Part model, mm, in its own coordinate system. A direction names the side the tool comes from. Round coordinates to 2 decimals unless told otherwise and drop trailing zeros. Answer as a JSON object with one key per item and string values. Group by question number.
from build123d import *

# Parameters (mm, degrees)
BOSS_EXTRUDE1_DEPTH = 4
BOSS_EXTRUDE1_TAPER = 10
CUT_EXTRUDE1_START  = 4
SKETCH1_3_R         = 1.1
CUT_EXTRUDE1_DEPTH  = 4
CUT_EXTRUDE2_START  = 4
SKETCH1_4_R         = 8.4
CUT_EXTRUDE2_DEPTH  = 3


with BuildPart() as part:
    # Sketch1 → Boss-Extrude1 (new body)
    with BuildSketch(Plane(origin=(0, 0, 0), x_dir=(1, 0, 0), z_dir=(0, 1, 0))):
        with BuildLine():
            ThreePointArc((-19.772689603, -11.447302995), (-15.6, -27.019992598), (-0.027310397, -22.847302995))
            Line((-0.027310397, -22.847302995), (9.872689603, -5.7))
            ThreePointArc((9.872689603, -5.7), (5.7, 9.872689603), (-9.872689603, 5.7))
            Line((-9.872689603, 5.7), (-19.772689603, -11.447302995))
        make_face()
    extrude(amount=BOSS_EXTRUDE1_DEPTH, taper=BOSS_EXTRUDE1_TAPER)

    # Sketch1<3> → Cut-Extrude1 (cut)
    with BuildSketch(Plane(origin=(0, 0, 0), x_dir=(1, 0, 0), z_dir=(0, 1, 0)).offset(CUT_EXTRUDE1_START)):
        with Locations(Location((-9.9, -17.147302995, 0), (0, 0, 270))):
            Circle(SKETCH1_3_R)
        with Locations(Location((0, 0, 0), (0, 0, 270))):
            Circle(SKETCH1_3_R)
    extrude(amount=-CUT_EXTRUDE1_DEPTH, mode=Mode.SUBTRACT)

    # Sketch1<4> → Cut-Extrude2 (cut)
    with BuildSketch(Plane(origin=(0, 0, 0), x_dir=(1, 0, 0), z_dir=(0, 1, 0)).offset(CUT_EXTRUDE2_START)):
        with Locations(Location((0, 0, 0), (0, 0, 270))):
            Circle(SKETCH1_4_R)
        with Locations(Location((-9.9, -17.147302995, 0), (0, 0, 270))):
            Circle(SKETCH1_4_R)
    extrude(amount=-CUT_EXTRUDE2_DEPTH, mode=Mode.SUBTRACT)


solid = part.part
Item 1: Which spindle directions (+Z, -Z, +X, -X, +Y, -Y) get a long thin tool onto all of the face, cutting with end or side? Do faces 1 (the face through (-9.531, 2.521, 8.755)), 2 (the face through (-10.6, 0.5, 16.3)). Say none if no direction does.
Item 2: Drop flat-ended pins along their axis: pin 1 Ø13.5 at (x, z) = (0, 0) entering from +Y; pin 2 Ø1 at (y, z) = (2.5, 5) entering from -X. Give the stop position or say it passes through.
Item 3: Band-saw the part on A-A, the plane y = 2.05. Count the separate pieces of the cut face and the enclosed holes in it, plus the area to 3 significant figures.
Item 4: Two-plate mould, pull along X, no slides. Class faces 3 (the face through (2.523, 2.521, 8.012)), 4 (the face through (-5, 4, 9)): pulls with the +X half, pulls with the -X half, needs draft (parallel to the pull), parting line crosses it, or undercut.
Item 5: Drill centre lines: line 1 (Z direction, x = 3, y = 3.2); line 2 (X direction, y = 1.8, z = 1.5); line 3 (X direction, y = 3.65, z = 7). Where is each one in solid material? Low to high.
Entries:
{
 "1": {"face 1": "+Y", "face 2": "+Y, -Y"},
 "2": {"pin 1": "y = 1", "pin 2": "x = -15.85"},
 "3": {"separate pieces": "1", "enclosed holes": "2", "area": "377 mm²"},
 "4": {"face 3": "undercut", "face 4": "needs draft"},
 "5": {"line 1": "-10.41 to -7.85, 7.85 to 16.48", "line 2": "-13.66 to -8.26, 8.26 to 10.98", "line 3": "-16.46 to -4.64, 4.64 to 8.38"}
}
